Autodesk Fusion 360 part; units mm, degrees
sketch "Counter holder" plane through (0, 0, 0) normal (0, 1, 0) x (1, 0, 0)
  line L0 (1.6795, -5.2373) -> (2.2579, -5.559)
  circle A0 centre (0, 0) radius 4.5
  line L1 (-1.6795, -5.2373) -> (-2.2579, -5.559)
  circle A1 centre (0, 0) radius 5.5
  arc A2 (2.2579, -5.559) -> (-1.5, 5.8095) centre (0, 0) ccw
  line L2 (0, 10.7) -> (-1.5, 10.7)
  line L3 (0, 10.7) -> (1.5, 10.7)
  arc A3 (-1.5, 5.8095) -> (-2.2579, -5.559) centre (0, 0) ccw
  line L4 (1.5, 10.7) -> (1.5, 5.8095)
  line L5 (-1.5, 10.7) -> (-1.5, 5.8095)
  point P0 (2.6505, 5.3709)
  dimension "d2" = 11
  dimension "d3" = 9
  dimension "d25" = 12
  dimension "d28" = 1.5
  dimension "d29" = 1.5
ref_plane "WorkPlane1" through (0, 10.85, 0) normal (0, 1, 0) x (1, 0, 0)
sketch "Servo holder" plane through (0, 10.85, 0) normal (0, 1, 0) x (1, 0, 0)
  circle A0 centre (0, 37.482) radius 3.5
  line L0 (0.0036, 26.913) -> (-1.4964, 26.913)
  line L1 (-1.4964, 26.913) -> (0.0036, 26.913)
  line L2 (0.0036, 26.913) -> (1.5036, 26.913)
  line L3 (1.5036, 26.913) -> (1.5036, 31.8089)
  line L4 (-1.4964, 26.913) -> (-1.4964, 31.807)
  arc A1 (-1.4964, 31.807) -> (1.5036, 31.8089) centre (0, 37.482) ccw
  arc A2 (1.5036, 31.8089) -> (-1.4964, 31.807) centre (0, 37.482) ccw
  point P0 (2.4711, 32.1586)
  point P1 (-2.4665, 32.1565)
  dimension "d6" = 11.738
  dimension "d7" = 7
  dimension "d31" = 1.5
  dimension "d32" = 1.5
extrude "Extrude4" add sketch "Counter holder" along normal blind 1 contours A1 makes body 1
extrude "Extrude5" add sketch "Counter holder" along normal blind 3 contours L0 L1 A1 A2 A3 bodies 1
extrude "Extrude6" add sketch "Counter holder" along normal blind 3 contours A2 L2 L3 L4 L5 bodies 1
extrude "Extrude7" add sketch "Servo holder" along normal blind 3 separate body contours A1 A2 makes body 2
extrude "Extrude8" add sketch "Servo holder" along normal blind 3 contours L0 L1 L2 L3 L4 A1 bodies 2
sketch "Connection" plane through (0, 0, 0) normal (1, 0, 0) x (0, 0, -1)
  line L0 (10.6742, 0.0115) -> (13.0212, 0.009) construction
  line L1 (13.0212, 0.009) -> (14.5207, 1.4657) construction
  line L2 (14.5207, 1.4657) -> (15.3617, 2.9367) construction
  line L3 (15.3617, 2.9367) -> (16.5492, 4.5723) construction
  line L4 (16.5492, 4.5723) -> (17.7004, 6.3241) construction
  line L5 (17.7004, 6.3241) -> (18.7215, 7.7387) construction
  line L6 (18.7215, 7.7387) -> (20.0559, 9.518) construction
  line L7 (20.0559, 9.518) -> (21.6526, 10.8269) construction
  line L8 (21.6526, 10.8269) -> (23.6966, 10.8532) construction
  line L9 (23.6966, 10.8532) -> (26.9817, 10.8544) construction
  spline S0 degree 5 poles (10.6742, 0.0115) (13.0212, 0.009) (14.5207, 1.4657) (15.3617, 2.9367) (16.5492, 4.5723) (17.7004, 6.3241) (18.7215, 7.7387) (20.0559, 9.518) (21.6526, 10.8269) (23.6966, 10.8532) (26.9817, 10.8544) knots 0 0 0 0 0 0 0.166667 0.333333 0.5 0.666667 0.833333 1 1 1 1 1 1
  spline S1 degree 5 poles (10.6774, 2.9747) (12.3316, 2.8904) (12.9969, 4.0027) (15.0793, 6.5355) (15.9956, 8.0056) (17.0271, 9.3169) (17.9968, 10.9661) (19.6323, 12.6073) (21.0727, 13.6625) (23.6453, 13.9834) (26.9849, 13.8452) knots 0 0 0 0 0 0 0.166667 0.333333 0.5 0.666667 0.833333 1 1 1 1 1 1
  line L10 (10.6774, 2.9747) -> (12.3316, 2.8904) construction
  line L11 (12.3316, 2.8904) -> (12.9969, 4.0027) construction
  line L12 (12.9969, 4.0027) -> (15.0793, 6.5355) construction
  line L13 (15.0793, 6.5355) -> (15.9956, 8.0056) construction
  line L14 (15.9956, 8.0056) -> (17.0271, 9.3169) construction
  line L15 (17.0271, 9.3169) -> (17.9968, 10.9661) construction
  line L16 (17.9968, 10.9661) -> (19.6323, 12.6073) construction
  line L17 (19.6323, 12.6073) -> (21.0727, 13.6625) construction
  line L18 (21.0727, 13.6625) -> (23.6453, 13.9834) construction
  line L19 (23.6453, 13.9834) -> (26.9849, 13.8452) construction
  line L20 (10.6774, 2.9747) -> (10.6742, 0.0115)
  line L21 (26.9849, 13.8452) -> (26.9817, 10.8544)
extrude "Extrude9" add sketch "Connection" along normal mid plane 3 bodies 1 2
Design review of the part built by this model. Coordinates are the model's own, in mm. A direction names the side the tool comes from. Round coordinates to 2 decimals unless told otherwise and drop trailing zeros. Write each loop counter-clockwise with the first axis right and the second up, starting at its lowest first coordinate (ties: lowest second). Pieces come first, ordered by that corner, then holes. Notation, with made-up numbers: (22.5, 27) -> (53.5, 27) arc R15 cw to (53.5, 41) -> close; hole circle Ø11 at (38, 25.25). An arc over 180 degrees is marked (long way). Write item = value, one per line. Start each with the question number.
1) Mouldability with a two-part tool opening along X and no side actions: class faces 1 (the face through (-5, 1, 0)), 2 (the face through (5.98, 1.48, -0.5)), 3 (the face through (0, 3, -6)) as +X half, -X half, draft (parallel to the pull), parting line (faces both ways), or undercut.
2) Take a section at A-A, the plane z = 0. State the section outline as (x, y) points, plus the area to 3 significant figures.
3) Wall thickness on probe 1 along X at (y, z) = (2.2, 0); probe 2 along X at (y, z) = (0.65, 0); probe 3 along Y at (x, z) = (0.25, -8): over which ranges is each line inside the solid? List them lowest first. Write a range as from..to.
4) Clearance check with flat-ended pins moving along their axes: pin 1 (6 mm diameter, centred on x = 2.5, z = -38, fed in from -Y); pin 2 (5 mm diameter, centred on x = -1.5, y = 11, fed in from +Z); pin 3 (3.5 mm diameter, centred on x = 1.5, z = -2.5, fed in from +Y). State where each tip first meets the part, or that it passes through.
5) Tool access review of faces 4 (the face through (-1.496, 12, -29)), 5 (the face through (0, 13.85, -33)), 6 (the face through (-0.218, 1.986, -5.496)), 7 (the face through (0, 10.85, -33)), 8 (the face through (1.504, 12, -29)): name each direction out of +Z, -Z, +X, -X, +Y, -Y from which nothing blocks a thin tool from reaching the whole face with its end or side.
Results list:
q1.face_1 = undercut
q1.face_2 = +X half
q1.face_3 = draft
q2.outline = (-6, 0) -> (-4.5, 0) -> (-4.5, 1) -> (-5.5, 1) -> (-5.5, 3) -> (-6, 3) -> close; (4.5, 0) -> (6, 0) -> (6, 3) -> (5.5, 3) -> (5.5, 1) -> (4.5, 1) -> close
q2.area = 5.00 mm²
q3.probe_1 = -6..-5.5, 5.5..6
q3.probe_2 = -6..-4.5, 4.5..6
q3.probe_3 = 0..3
q4.pin_1 = 10.85
q4.pin_2 = -16.39
q4.pin_3 = 1
q5.face_4 = +Z, -X, +Y, -Y
q5.face_5 = -Z, +X, -X, +Y
q5.face_6 = +Y
q5.face_7 = -Z, +X, -X, -Y
q5.face_8 = +Z, +X, +Y, -Y
